from build123d import *

# Parameters (mm, degrees)
SKETCH1_W                    = 26.3
SKETCH1_H                    = 10
BASE_FLANGE1_DEPTH           = 0.5
EDGE_FLANGE1_STRIP_W         = 2.3
EDGE_FLANGE1_STRIP_H         = 0.5
EDGE_FLANGE1_STRIP_CUT_DEPTH = 10
EDGE_FLANGE1_DEPTH           = 10
EDGE_FLANGE1_PROFILE_W       = 16
EDGE_FLANGE1_PROFILE_H       = 8.35
EDGE_FLANGE1_FLAT_DEPTH      = 0.5
M4_START                     = -0.5
M4_CLEARANCE_SLOT1_DEPTH     = 0.5


# Read off the part's stored shape, not the designer's step: M4 Clearance Slot1
# Sheet-metal steps are written as plain solids
with BuildPart() as part:
    # Sketch1 → Base-Flange1 (new body)
    with BuildSketch(Plane.XY):
        with Locations((13.15, 0)):
            Rectangle(SKETCH1_W, SKETCH1_H)
    extrude(amount=-BASE_FLANGE1_DEPTH)

    # Edge-Flange1 strip (across the edge) → Edge-Flange1 strip cut (cut)
    with BuildSketch(Plane(origin=(26.3, -5, 0), x_dir=(-1, 0, 0), z_dir=(0, 1, 0))):
        with Locations((-0.5, -0.25)):
            Rectangle(EDGE_FLANGE1_STRIP_W, EDGE_FLANGE1_STRIP_H)
    extrude(amount=EDGE_FLANGE1_STRIP_CUT_DEPTH, mode=Mode.SUBTRACT)

    # Edge-Flange1 bend section (across the edge) → Edge-Flange1 (add)
    with BuildSketch(Plane(origin=(26.3, -5, 0), x_dir=(-1, 0, 0), z_dir=(0, 1, 0))):
        with BuildLine():
            Line((0, 0.15), (0.5, 0.15))
            ThreePointArc((0.5, 0.15), (0.543933983, 0.043933983), (0.65, 0))
            Line((0.65, 0), (0.65, -0.5))
            ThreePointArc((0.65, -0.5), (0.190380592, -0.309619408), (0, 0.15))
        make_face()
    extrude(amount=EDGE_FLANGE1_DEPTH)

    # Edge-Flange1 profile (on flange) → Edge-Flange1 flat (add)
    with BuildSketch(Plane.YZ.offset(26.3)):
        with Locations((0, 4.325)):
            Rectangle(EDGE_FLANGE1_PROFILE_W, EDGE_FLANGE1_PROFILE_H)
    extrude(amount=-EDGE_FLANGE1_FLAT_DEPTH)

    # M4 Clearance Slot1 outline → M4 Clearance Slot1 (cut)
    with BuildSketch(Plane.XY.offset(M4_START)):
        with BuildLine():
            Line((14, -1.040099885), (14, 1.040099885))
            ThreePointArc((14, 1.040099885), (11.75, 3.290099885), (9.5, 1.040099885))
            Line((9.5, 1.040099885), (9.5, -1.040099885))
            ThreePointArc((9.5, -1.040099885), (11.75, -3.290099885), (14, -1.040099885))
        make_face()
        with BuildLine():
            Line((6.75, -1.040099885), (6.75, 1.040099885))
            ThreePointArc((6.75, 1.040099885), (4.5, 3.290099885), (2.25, 1.040099885))
            Line((2.25, 1.040099885), (2.25, -1.040099885))
            ThreePointArc((2.25, -1.040099885), (4.5, -3.290099885), (6.75, -1.040099885))
        make_face()
    extrude(amount=M4_CLEARANCE_SLOT1_DEPTH, mode=Mode.SUBTRACT)


solid = part.part
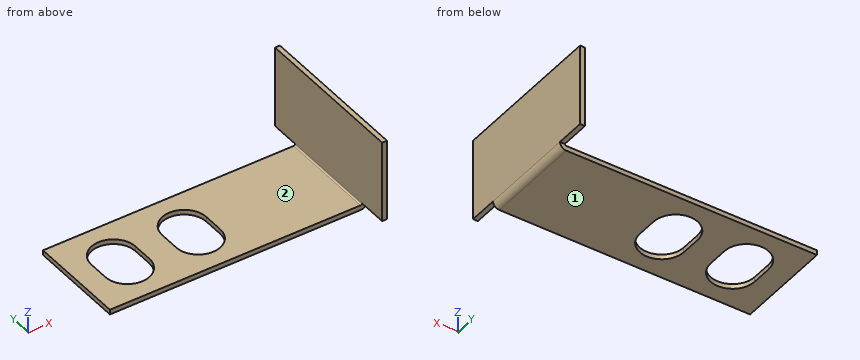
Work out the finished part from the listing and answer in its coordinate system (mm). Face numbers are marked on the shaded views. A direction names the side the tool comes from. Give positions to 0.01 mm unless a question says otherwise; leave off trailing zeros. Write each loop counter-clockwise with the first axis right and the second up, starting at its lowest first coordinate (ties: lowest second). Pieces come first, ordered by that corner, then holes. Notation, with made-up numbers: (56, 36.25) - (92, 36.25) arc R17 ccw to (92, 45.25) - close; hole circle Ø1 at (-27, 0.5). An arc over 180 degrees is marked (long way). One line per item, written item: value. Start each with the question number.
1. Find section A-A (x = 4.5). Write down the section's boundary in (y, z), then the cut area to 3 significant figures.
2. Find section C-C (y = -3.75). Write down the section's boundary in (x, z).
3. Given pin 1 (1 mm diameter, centred on x = 19.5, y = 5, fed in from +Z); pin 2 (5 mm diameter, centred on y = -1, z = 4.5, fed in from -X); pin 3 (0.6 mm diameter, centred on x = 26, y = -6, fed in from -Z); pin 4 (2 mm diameter, centred on x = 11, z = 2.5, fed in from +Y), each flat-ended and moving along its own axis, determine where each tip first touches the part or whether it passes through.
4. Find section B-B (y = 2.25). Write down the section's boundary in (x, z), then the cut area to 3 significant figures.
5. Consider probe 1 along X at (y, z) = (3.75, 2.75); probe 2 along Z at (x, y) = (13.5, -4.5). Determine where each line is inside the solid, lowest interval first.
6. Find section D-D (x = 10). Write down the section's boundary in (y, z), then the cut area to 3 significant figures.
7. For the marked faces 1 and 2, determine the directions among +Z, -Z, +X, -X, +Y, -Y from which every point of the face is accessible in a straight line to the end or side of a thin tool.
Geometry results:
1. outline: (-5, -0.5) - (-3.29, -0.5) - (-3.29, 0) - (-5, 0) - close; (3.29, -0.5) - (5, -0.5) - (5, 0) - (3.29, 0) - close
1. area: 1.71 mm2
2. outline: (0, -0.5) - (25.65, -0.5) arc R0.65 ccw to (26.3, 0.15) - (26.3, 8.5) - (25.8, 8.5) - (25.8, 0.15) arc R0.15 cw to (25.65, 0) - (0, 0) - close
3. pin 1: z = 0
3. pin 2: x = 25.8
3. pin 3: z = 0.15
3. pin 4: through
4. outline: (0, -0.5) - (2.6, -0.5) - (2.6, 0) - (0, 0) - close; (6.4, -0.5) - (9.85, -0.5) - (9.85, 0) - (6.4, 0) - close; (13.65, -0.5) - (25.65, -0.5) arc R0.65 ccw to (26.3, 0.15) - (26.3, 8.5) - (25.8, 8.5) - (25.8, 0.15) arc R0.15 cw to (25.65, 0) - (13.65, 0) - close
4. area: 13.5 mm2
5. probe 1: 25.8 to 26.3
5. probe 2: -0.5 to 0
6. outline: (-5, -0.5) - (-2.45, -0.5) - (-2.45, 0) - (-5, 0) - close; (2.45, -0.5) - (5, -0.5) - (5, 0) - (2.45, 0) - close
6. area: 2.55 mm2
7. face 1: -Z, +X, -X, +Y, -Y
7. face 2: +Z, -X, +Y, -Y
